Can you work these out from the model? Positions are in its coordinate system, mm. A direction names the side the tool comes from. Coordinates: 2 decimals unless noted, no trailing zeros. Loops run counter-clockwise (first coordinate to the right, second up) from the corner with the lowest first, then second, coordinate; pieces in that order, holes last. Notation, with made-up numbers: (12, -15) -> (50, -15) arc R25 ccw to (50, 16) -> close; hole circle Ø3 at (-35, 66.25). An arc over 180 degrees is marked (long way). Put each result on its own line as item: value. Start each with the question number.
Item 1: Please list where these lines run through material, in increasing order: L1, parallel to Y at x = -32, z = 2.5; L2, parallel to X at y = -16, z = -48.5; L3, parallel to X at y = -4, z = -27. Write a range as from..to.
Item 2: If we section it at A-A on y = -18: Please give me the cut outline in (x, z), plus the area to 3 significant figures.
Item 3: For faces 5 (the cylindrical face through (-45, -16, -52)), 6 (the flat face through (-29, -15, -72)), 7 (the flat face through (-34.7, 41.3, -5)), 8 (the cylindrical face through (-32.45, 2.85, -3.01)), which set-ups out of +Z, -Z, +X, -X, +Y, -Y let a thin tool reach every point of the face, with its end or its side?
Item 4: We'd pull the mould along X, two halves only. Please class faces 1 (the flat face through (-64, -9, -15)), 2 (the flat face through (-49, -18, -77)), 3 (the flat face through (0, -9, -15)), 4 (the flat face through (-35, -12, -26)): pulls with the +X half, pulls with the -X half, needs draft (parallel to the pull), parting line crosses it, or undercut.
Item 5: If we section it at D-D on z = -69: Please give me the cut outline in (x, y).
Item 6: Will these pins go through, and if not, where does the flat tip stop? P1, Ø12, axis at x = -33.5, z = -23, coming from the -Y side; P2, Ø5, axis at x = -43, z = -21, coming from the +Y side; P3, Ø16, axis at x = -31.5, y = 46, coming from the -Z side; P4, Ø1, axis at x = -19.5, z = 10, coming from the +Y side.
Item 7: If we section it at B-B on z = -18: Please give me the cut outline in (x, y), plus the area to 3 significant figures.
```python
from build123d import *

# Parameters (mm, degrees)
ESTRUSIONE_ESTRUSIONE1_DEPTH = 64
RACCORDO1_RADIUS             = 32
RACCORDO1_LENGTH             = 25
SCHIZZO2_R                   = 13
TAGLIO_ESTRUSIONE1_DEPTH     = 119.831813922
SCHIZZO5_W                   = 6
SCHIZZO5_H                   = 64
TAGLIO_ESTRUSIONE2_DEPTH     = 119.831813922
TAGLIO_ESTRUSIONE3_DEPTH     = 119.831813922
SCHIZZO7_R                   = 3
TAGLIO_ESTRUSIONE4_DEPTH     = 119.831813922
SCHIZZO8_R                   = 12.5
ESTRUSIONE_ESTRUSIONE2_DEPTH = 5
SCHIZZO9_R                   = 9.5
TAGLIO_ESTRUSIONE5_DEPTH     = 116.654658358
RACCORDO2_R                  = 10
RACCORDO3_R                  = 5


with BuildPart() as part:
    # Schizzo1 → Estrusione-Estrusione1 (new body)
    with BuildSketch(Plane(origin=(0, 0, 0), x_dir=(0, 0, -1), z_dir=(1, 0, 0))):
        Polygon((0, 0), (77, 0), (77, -25), (-25, -25), (-25, 64), (0, 64), align=None)
    extrude(amount=-ESTRUSIONE_ESTRUSIONE1_DEPTH)

    # Raccordo1: full round fillet: the end face becomes a half cylinder, R = half its width
    raccordo1_face = Plane((-32, 64, 12.5), x_dir=(0, 0, -1), z_dir=(0, 1, 0))  # on the end face: x along it, z out of the body
    raccordo1_slab = raccordo1_face.offset(-RACCORDO1_RADIUS / 2) * Box(RACCORDO1_LENGTH, 2 * RACCORDO1_RADIUS, RACCORDO1_RADIUS, mode=Mode.PRIVATE)  # the body's end, R deep
    raccordo1_round = Plane((-32, 32, 12.5), x_dir=(0, 1, 0), z_dir=(0, 0, -1)) * Cylinder(RACCORDO1_RADIUS, RACCORDO1_LENGTH, mode=Mode.PRIVATE)  # its axis R under the face
    add(raccordo1_slab - raccordo1_round, mode=Mode.SUBTRACT)

    # Schizzo2 → Taglio-Estrusione1 (cut, through all)
    with BuildSketch(Plane(origin=(0, 0, 0), x_dir=(1, 0, 0), z_dir=(0, 1, 0))):
        with Locations(Location((-32, 52, 0), (0, 0, 270))):
            Circle(SCHIZZO2_R)
    extrude(amount=-TAGLIO_ESTRUSIONE1_DEPTH, mode=Mode.SUBTRACT)

    # Schizzo5 → Taglio-Estrusione2 (cut, through all)
    with BuildSketch(Plane(origin=(0, 0, 0), x_dir=(1, 0, 0), z_dir=(0, 1, 0))):
        with Locations((-32, 45)):
            Rectangle(SCHIZZO5_W, SCHIZZO5_H)
    extrude(amount=-TAGLIO_ESTRUSIONE2_DEPTH, mode=Mode.SUBTRACT)

    # Schizzo6 → Taglio-Estrusione3 (cut, through all)
    with BuildSketch(Plane(origin=(0, 0, 0), x_dir=(0, 0, -1), z_dir=(1, 0, 0))):
        Polygon((26, 0), (77, -12), (77, 0), align=None)
    extrude(amount=-TAGLIO_ESTRUSIONE3_DEPTH, mode=Mode.SUBTRACT)

    # Schizzo7 → Taglio-Estrusione4 (cut, through all)
    with BuildSketch(Plane(origin=(0, 0, 0), x_dir=(0, 0, -1), z_dir=(1, 0, 0))):
        with Locations((70, -18)):
            Circle(SCHIZZO7_R)
    extrude(amount=-TAGLIO_ESTRUSIONE4_DEPTH, mode=Mode.SUBTRACT)

    # Schizzo8 → Estrusione-Estrusione2 (add)
    with BuildSketch(Plane(origin=(0, 0, 0), x_dir=(-1, 0, 0), z_dir=(0, 0, -1))):
        with Locations((32, 32)):
            Circle(SCHIZZO8_R)
    extrude(amount=ESTRUSIONE_ESTRUSIONE2_DEPTH)

    # Schizzo9 → Taglio-Estrusione5 (cut, through all)
    with BuildSketch(Plane(origin=(0, 0, -5), x_dir=(-1, 0, 0), z_dir=(0, 0, -1))):
        with Locations((32, 32)):
            Circle(SCHIZZO9_R)
    extrude(amount=-TAGLIO_ESTRUSIONE5_DEPTH, mode=Mode.SUBTRACT)

    # Raccordo2
    raccordo2_edges = [part.edges().sort_by_distance(p)[0] for p in [
        (-32, 0, 0),
    ]]
    fillet(raccordo2_edges, radius=RACCORDO2_R)

    # Raccordo3
    raccordo3_edges = [part.edges().sort_by_distance(p)[0] for p in [
        (-19.5, 32, 0),
    ]]
    fillet(raccordo3_edges, radius=RACCORDO3_R - 0.0001)  # a hair under: the kernel refuses the full size


solid = part.part
```
Solutions:
1. L1: -25..22.5, 41.5..64
1. L2: -64..-44.52, -19.48..0
1. L3: -64..-35, -29..0
2. outline: (-64, -77) -> (-35, -77) -> (-35, -73) -> (-64, -73) -> close; (-64, -67) -> (-35, -67) -> (-35, -64.65) arc R13 cw to (-35, -39.35) -> (-35, -13) -> (-29, -13) -> (-29, -39.35) arc R13 cw to (-29, -64.65) -> (-29, -67) -> (0, -67) -> (0, 25) -> (-64, 25) -> close; (-29, -77) -> (0, -77) -> (0, -73) -> (-29, -73) -> close
2. area: 5,420 mm^2
3. face 5: +Y, -Y
3. face 6: -Z, +Y, -Y
3. face 7: -Z, +X, -X, +Y
3. face 8: -Z, +X, -X
4. face 1: pulls with the -X half
4. face 2: needs draft
4. face 3: pulls with the +X half
4. face 4: undercut
5. outline: (-64, -25) -> (-35, -25) -> (-35, -20.83) -> (-64, -20.83) -> close; (-64, -15.17) -> (-35, -15.17) -> (-35, -10.12) -> (-64, -10.12) -> close; (-29, -25) -> (0, -25) -> (0, -20.83) -> (-29, -20.83) -> close; (-29, -15.17) -> (0, -15.17) -> (0, -10.12) -> (-29, -10.12) -> close
6. P1: y = -25
6. P2: y = 0
6. P3: z = -5
6. P4: y = 61.66
7. outline: (-64, -25) -> (-35, -25) -> (-35, 0) -> (-64, 0) -> close; (-29, -25) -> (0, -25) -> (0, 0) -> (-29, 0) -> close
7. area: 1,450 mm^2
